```python
from build123d import *

# Parameters (mm, degrees)
BOSS_EXTRUDE2_DEPTH = 7
SKETCH3_R           = 0.5
CUT_EXTRUDE3_DEPTH  = 8.842193571


with BuildPart() as part:
    # Sketch1 → Boss-Extrude2 (new body)
    with BuildSketch(Plane(origin=(0, 0, 0), x_dir=(1, 0, 0), z_dir=(0, 1, 0))):
        with BuildLine():
            Line((-2.5, 0), (2.5, 0))
            ThreePointArc((2.5, 0), (0, -2.5), (-2.5, 0))
        make_face()
    extrude(amount=BOSS_EXTRUDE2_DEPTH)

    # Sketch3 → Cut-Extrude3 (cut, through all)
    with BuildSketch(Plane(origin=(0, 0, 0), x_dir=(1, 0, 0), z_dir=(0, 1, 0))):
        with Locations((-2.5, 0)):
            Circle(SKETCH3_R)
        with Locations((-1.741766773, -1.793390227)):
            Circle(SKETCH3_R)
        with Locations((0.072998806, -2.498934008)):
            Circle(SKETCH3_R)
        with Locations((1.843484289, -1.688657951)):
            Circle(SKETCH3_R)
        with Locations((2.495736939, 0.145935359)):
            Circle(SKETCH3_R)
    extrude(amount=CUT_EXTRUDE3_DEPTH, mode=Mode.SUBTRACT)


solid = part.part
```
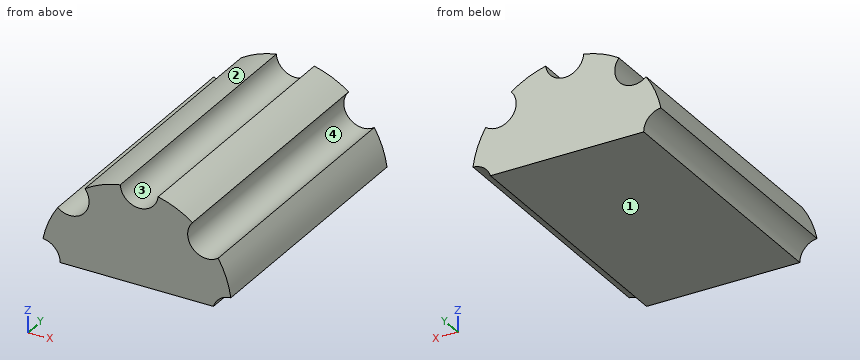
Verification items for the finished model (mm, model axes). Face numbers are marked on the shaded views. Round coordinates to 2 decimals unless told otherwise and drop trailing zeros. Loops run counter-clockwise (first coordinate to the right, second up) from the corner with the lowest first, then second, coordinate; pieces in that order, holes last. Notation, with made-up numbers: (69.25, 51.5) -> (82.25, 51.5) arc R17 cw to (82.25, 63.5) -> close; hole circle Ø2 at (-5.5, 41.25). An arc over 180 degrees is marked (long way). Answer as a JSON object with one key per item and string values.
Q1. Section check B-B (z = 0.7). Record the boundary of the cut face in (x, y).
Data:
{"outline": "(-2.4, 0) -> (2.4, 0) -> (2.4, 7) -> (-2.4, 7) -> close"}
Q2. Go/stop test with a flat-tipped pin: P1, Ø1, axis at y = 1, z = 1.5, coming from the -X side. Record where the tip stops, or that it passes through.
Data:
{"P1": "stops at x = -2.29"}
Q3. Section check A-A (y = 2.75). Record the boundary of the cut face in (x, z).
Data:
{"outline": "(-2.45, 0.5) arc R0.5 cw to (-2, 0) -> (2.02, 0) arc R0.5 cw to (2.47, 0.35) arc R2.5 ccw to (2.14, 1.29) arc R0.5 cw to (1.47, 2.02) arc R2.5 ccw to (0.57, 2.43) arc R0.5 cw to (-0.43, 2.46) arc R2.5 ccw to (-1.35, 2.1) arc R0.5 cw to (-2.06, 1.41) arc R2.5 ccw to start"}
Q4. Section check C-C (x = 1.85). Record the boundary of the cut face in (y, z).
Data:
{"outline": "(0, 0) -> (7, 0) -> (7, 1.19) -> (0, 1.19) -> close"}
Q5. Scan lines: line 1 (X direction, y = 5, z = 2.25); line 2 (Z direction, x = -1.7, y = 5.25); line 3 (Z direction, x = -0.9, y = 4). Record each from-to range of solid material in increasing order. Write a range as from..to.
Data:
{"line 1": "x = -1.09..-0.36, 0.51..1.09", "line 2": "z = 0..1.3", "line 3": "z = 0..2.33"}
Q6. Draft check along X on the marked faces 1, 2, 3 and 4. Enter one of: pulls with the +X half, pulls with the -X half, needs draft (parallel to the pull), parting line crosses it, or undercut.
Data:
{"face 1": "needs draft", "face 2": "pulls with the -X half", "face 3": "undercut", "face 4": "undercut"}
